```python
from build123d import *

# Parameters (mm, degrees)
BOSS_EXTRUDE1_DEPTH = 76.2
CUT_EXTRUDE1_DEPTH  = 173.688654555
BOSS_EXTRUDE2_DEPTH = 5.334


with BuildPart() as part:
    # Sketch4 → Boss-Extrude1 (new, symmetric)
    with BuildSketch(Plane(origin=(0, 0, 0), x_dir=(1, 0, 0), z_dir=(0, 1, 0))):
        Polygon((57.426524411, 0), (56.323089847, 11.20335914), (53.055190527, 21.976179471), (47.748409988, 31.904467549), (40.606684831, 40.606684831), (31.904467549, 47.748409988), (21.976179471, 53.055190527), (11.20335914, 56.323089847), (0, 57.426524411), (-11.20335914, 56.323089847), (-21.976179471, 53.055190527), (-31.904467549, 47.748409988), (-40.606684831, 40.606684831), (-47.748409988, 31.904467549), (-53.055190527, 21.976179471), (-56.323089847, 11.20335914), (-57.426524411, 0), (-56.323089847, -11.20335914), (-53.055190527, -21.976179471), (-47.748409988, -31.904467549), (-40.606684831, -40.606684831), (-31.904467549, -47.748409988), (-21.976179471, -53.055190527), (-11.20335914, -56.323089847), (0, -57.426524411), (11.20335914, -56.323089847), (21.976179471, -53.055190527), (31.904467549, -47.748409988), (40.606684831, -40.606684831), (47.748409988, -31.904467549), (53.055190527, -21.976179471), (56.323089847, -11.20335914), align=None)
    extrude(amount=BOSS_EXTRUDE1_DEPTH, both=True)

    # Sketch5 → Cut-Extrude1 (cut, through all)
    with BuildSketch(Plane(origin=(0, 76.2, 0), x_dir=(1, 0, 0), z_dir=(0, 1, 0))):
        Polygon((51.316592972, -10.207504994), (52.321944464, 0), (51.316592972, 10.207504994), (48.339173591, 20.022741295), (43.504106878, 29.068514878), (36.997201735, 36.997201735), (29.068514878, 43.504106878), (20.022741295, 48.339173591), (10.207504994, 51.316592972), (0, 52.321944464), (-10.207504994, 51.316592972), (-20.022741295, 48.339173591), (-29.068514878, 43.504106878), (-36.997201735, 36.997201735), (-43.504106878, 29.068514878), (-48.339173591, 20.022741295), (-51.316592972, 10.207504994), (-52.321944464, 0), (-51.316592972, -10.207504994), (-48.339173591, -20.022741295), (-43.504106878, -29.068514878), (-36.997201735, -36.997201735), (-29.068514878, -43.504106878), (-20.022741295, -48.339173591), (-10.207504994, -51.316592972), (0, -52.321944464), (10.207504994, -51.316592972), (20.022741295, -48.339173591), (29.068514878, -43.504106878), (36.997201735, -36.997201735), (43.504106878, -29.068514878), (48.339173591, -20.022741295), align=None)
    extrude(amount=-CUT_EXTRUDE1_DEPTH, mode=Mode.SUBTRACT)

    # Sketch6 → Boss-Extrude2 (add)
    with BuildSketch(Plane.XZ.offset(76.2)):
        Polygon((-51.316592972, 10.207504994), (-52.321944464, 0), (-57.377482875, 0.497927073), (-56.372131384, 10.705432067), align=None)
        Polygon((57.377482875, -0.497927073), (56.372131384, -10.705432067), (51.316592972, -10.207504994), (52.321944464, 0), align=None)
        Polygon((-47.748409988, -31.904467549), (-40.606684831, -40.606684831), (-36.679791728, -37.383966948), (-43.821516885, -28.681749665), align=None)
        Polygon((36.997201735, -36.997201735), (29.068514878, -43.504106878), (32.291232761, -47.430999981), (40.219919619, -40.924094838), align=None)
        Polygon((47.430999981, 32.291232761), (40.924094838, 40.219919619), (36.997201735, 36.997201735), (43.504106878, 29.068514878), align=None)
        Polygon((-37.383966948, 36.679791728), (-28.681749665, 43.821516885), (-31.904467549, 47.748409988), (-40.606684831, 40.606684831), align=None)
        Polygon((0, 52.321944464), (10.207504994, 51.316592972), (10.705432067, 56.372131384), (0.497927073, 57.377482875), align=None)
        Polygon((-10.705432067, -56.372131384), (-0.497927073, -57.377482875), (0, -52.321944464), (-10.207504994, -51.316592972), align=None)
    extrude(amount=BOSS_EXTRUDE2_DEPTH)


solid = part.part
```
The listing builds one solid part. Answer for the finished solid, in the listing's coordinates (mm). A direction names the side the tool comes from. Give positions to 0.01 mm unless a question says otherwise; leave off trailing zeros. Write each loop counter-clockwise with the first axis right and the second up, starting at its lowest first coordinate (ties: lowest second). Pieces come first, ordered by that corner, then holes. Notation, with made-up numbers: (1, -20.75) -> (9, -20.75) arc R21 ccw to (9, 1.25) -> close; hole circle Ø7 at (0.5, -12). An arc over 180 degrees is marked (long way). Write item = value, one per line. Start each with the question number.
1) Straight lines are drawn through the part: line 1 along Z through (x, y) = (-8.5, -54.5); line 2 along X through (y, z) = (-45.5, 19.5); line 3 along Z through (x, y) = (15, -20.5). For each, find the intervals that lie inside material, in ascending order.
2) The part is cut by section B-B, the plane z = 7.5. Determine the outline of the cut face in (x, y), and give its area (3 significant figures).
3) Determine the mould class of faces 4 (the face through (-45.888, 1.067, -24.609)), 5 (the face through (54.712, 1.067, -16.514)), 6 (the face through (-36.316, -1.563, 44.128)) for opening direction Z: +Z half, -Z half, draft (parallel to the pull), parting line (faces both ways), or undercut.
4) The part is cut by section A-A, the plane x = -34.5. Determine the outline of the cut face in (y, z), and give its area (3 significant figures).
5) Each of these flat-tipped pins is pushed along its axis until it touches: pin 1 (11 mm diameter, centred on x = -50, z = -19, fed in from -Y); pin 2 (21.5 mm diameter, centred on x = -18, z = -49.5, fed in from -Y); pin 3 (4 mm diameter, centred on y = -19, z = 13, fed in from +X); pin 4 (4 mm diameter, centred on y = 7, z = -43.5, fed in from -X). Where does it stop, or does it pass through?
6) Which of the six approach directions +Z, -Z, +X, -X, +Y, -Y give full straight-line access (tool end or side, diameter ignored) to faces 1 (the face through (-44.23, 1.07, 36.19)), 2 (the face through (40.205, -1.563, 33.088)), 3 (the face through (38.988, -78.83, 38.631))?
Solutions:
q1.line_1 = -56.59 to -51.48, 51.48 to 56.59
q1.line_2 = -53.81 to -48.5, 48.5 to 53.81
q1.line_3 = -55.17 to -49.86, 49.86 to 55.17
q2.outline = (-56.69, -81.53) -> (-51.58, -81.53) -> (-51.58, 76.2) -> (-56.69, 76.2) -> close; (51.58, -76.2) -> (56.69, -76.2) -> (56.69, 76.2) -> (51.58, 76.2) -> close
q2.area = 1,580 mm²
q3.face_4 = undercut
q3.face_5 = -Z half
q3.face_6 = +Z half
q4.outline = (-81.53, 39.05) -> (76.2, 39.05) -> (76.2, 45.62) -> (-81.53, 45.62) -> close; (-76.2, -45.62) -> (76.2, -45.62) -> (76.2, -39.05) -> (-76.2, -39.05) -> close
q4.area = 2,040 mm²
q5.pin_1 = -76.2
q5.pin_2 = -81.53
q5.pin_3 = 56.34
q5.pin_4 = -39.52
q6.face_1 = +Z, -X, +Y, -Y
q6.face_2 = +Y, -Y
q6.face_3 = +Z, -Y
